Design review of the part built by this model. Coordinates are the model's own, in mm. A direction names the side the tool comes from. Round coordinates to 2 decimals unless told otherwise and drop trailing zeros. Order: outer loops, then holes, each group sorted by start corner. A loop starts at its lowest first (then second) coordinate and runs counter-clockwise, first axis right, second up. Notation, with made-up numbers: (-9.75, -21) - (40.25, -21) arc R15 cw to (40.25, 4) - close; hole circle Ø10 at (77.25, 1). An arc over 180 degrees is marked (long way). Use CSV: the item, a comma, the result in double quotes. Start each with the question number.
Autodesk Inventor part; units mm, degrees
ref_plane "YZ Plane" through (0, 0, 0) normal (1, 0, 0) x (0, 1, 0)
ref_plane "XZ Plane" through (0, 0, 0) normal (0, 1, 0) x (-1, 0, 0)
ref_plane "XY Plane" through (0, 0, 0) normal (0, 0, 1) x (1, 0, 0)
sketch "Sketch1" plane through (0, 0, 0) normal (0, 1, 0) x (-1, 0, 0)
  line L0 (0, 0) -> (20, 0)
  line L1 (20, 0) -> (20, 30)
  line L2 (20, 30) -> (0, 30)
  line L3 (0, 30) -> (0, 0)
  line L4 (0, 30) -> (20, 0)
  line L5 (0, 0) -> (20, 30)
  line L6 (11.5, 3.5) -> (8.5, 3.5)
  line L7 (3.5, 8.5) -> (3.5, 21.5)
  line L8 (8.5, 26.5) -> (11.5, 26.5)
  line L9 (16.5, 21.5) -> (16.5, 8.5)
  line L10 (16.5, 3.5) -> (3.5, 26.5) construction
  line L11 (3.5, 3.5) -> (16.5, 26.5) construction
  arc A0 (8.5, 26.5) -> (3.5, 21.5) centre (8.5, 21.5) ccw
  arc A1 (16.5, 21.5) -> (11.5, 26.5) centre (11.5, 21.5) ccw
  arc A2 (11.5, 3.5) -> (16.5, 8.5) centre (11.5, 8.5) ccw
  arc A3 (3.5, 8.5) -> (8.5, 3.5) centre (8.5, 8.5) ccw
  line L12 (12.5954, 0) -> (7.0954, 0)
  line L13 (7.0954, 0) -> (7.0954, 1.5)
  line L14 (7.0954, 1.5) -> (12.5954, 1.5)
  line L15 (12.5954, 1.5) -> (12.5954, 0)
  point P0 (10, 15)
  dimension "d0" = 20
  dimension "d1" = 30
  dimension "d5" = 13
  dimension "d6" = 23
  dimension "d7" = 5
  dimension "d10" = 5.5
  dimension "d11" = 1.5
extrude "Extrusion1" add sketch "Sketch1" along normal blind 5
fillet "Fillet1" radius 10 4 edges at (0, 2.5, 30) (0, 2.5, 0) (-20, 2.5, 0) (-20, 2.5, 30)
extrude "Extrusion2" cut sketch "Sketch1" along normal blind 1 contours A3 L7 A0 L4 L5 | L5 L4 A2 L6 A3 | A0 L8 A1 L5 L4 | L5 A1 L9 A2 L4
properties part number "glosnik"
Q1. Take a section at D-D (z = 27.5). State the section outline as (x, y) points, plus the area to 3 significant figures.
Q2. Take a section at C-C (x = -4). State the section outline as (y, z) points, plus the area to 3 significant figures.
Q3. Tool access review of faces 1 (the flat face through (0, 2, 15)), 2 (the flat face through (-10, 0.5, 3.5)): name each direction out of +Z, -Z, +X, -X, +Y, -Y from which nothing blocks a thin tool from reaching the whole face with its end or side.
Q4. For L1, parallel to Y at x = -9.5, z = 11.5; L2, parallel to X at y = 0.7, z = 8.5; L3, parallel to Z at x = -14.5, y = 0.7, list the stretches that pass through material, from the lowest coordinate up. Write a range as [from, to].
Q5. Clearance check with flat-ended pins moving along their axes: pin 1 (6.5 mm diameter, centred on x = -7.5, z = 15.5, fed in from -Y); pin 2 (2 mm diameter, centred on x = -15.5, y = 1, fed in from -Z). State where each tip first meets the part, or that it passes through.
Q6. The part is to be moulded in two halves that separate along X. For faces 3 (the cylindrical face through (-17.15, 2.54, 26.99)), 4 (the cylindrical face through (-2.85, 2.54, 3.01)), 5 (the cylindrical face through (-5, 0.49, 4.93)), say which applies: +X half, -X half, draft (parallel to the pull), parting line (faces both ways), or undercut.
Q7. Take a section at B-B (z = 15). State the section outline as (x, y) points.
Findings below:
1,outline,"(-16.61, 0) - (-3.39, 0) - (-3.39, 5) - (-16.61, 5) - close"
1,area,"66.1 mm^2"
2,outline,"(0, 2) - (5, 2) - (5, 28) - (0, 28) - (0, 23.68) - (1, 23.68) - (1, 6.32) - (0, 6.32) - close"
2,area,"113 mm^2"
3,face 1,"+Z, -Z, +X, +Y, -Y"
3,face 2,"-Y"
4,L1,"y = [1, 5]"
4,L2,"x = [-19.89, -16.5], [-3.5, -0.11]"
4,L3,"z = [1.07, 4.5], [25.5, 28.93]"
5,pin 1,"stops at y = 1"
5,pin 2,"stops at z = 1.07"
6,face 3,"-X half"
6,face 4,"+X half"
6,face 5,"undercut"
7,outline,"(-20, 0) - (-16.5, 0) - (-16.5, 1) - (-3.5, 1) - (-3.5, 0) - (0, 0) - (0, 5) - (-20, 5) - close"
